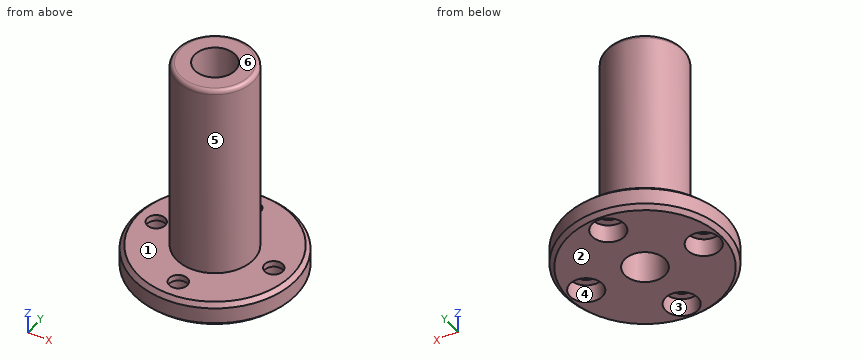
```python
from build123d import *

# Parameters (mm, degrees)
F0_R     = 20
F0_R_2   = 2.25
F0_R_3   = 5
F1_DEPTH = 6
F2_R     = 9.5
F2_R_2   = 5
F3_DEPTH = 49
F4_R     = 4
F5_DEPTH = 4.5
F6_SIZE  = 1
F7_R     = 1


with BuildPart() as f1:
    # F0 (on Top) → F1 (new body)
    with BuildSketch(Plane.XY):
        Circle(F0_R)
        with Locations((0, -14.5)):
            Circle(F0_R_2, mode=Mode.SUBTRACT)
        with Locations((-14.5, 0)):
            Circle(F0_R_2, mode=Mode.SUBTRACT)
        Circle(F0_R_3, mode=Mode.SUBTRACT)
        with Locations((14.5, 0)):
            Circle(F0_R_2, mode=Mode.SUBTRACT)
        with Locations((0, 14.5)):
            Circle(F0_R_2, mode=Mode.SUBTRACT)
    extrude(amount=F1_DEPTH)

    # F2 (on face) → F3 (join)
    with BuildSketch(Plane.XY.offset(6)):
        Circle(F2_R)
        Circle(F2_R_2, mode=Mode.SUBTRACT)
    extrude(amount=F3_DEPTH)

    # F4 (on face) → F5 (cut)
    with BuildSketch(Plane(origin=(0, 0, 0), x_dir=(1, 0, 0), z_dir=(0, 0, -1))):
        with Locations((0, 14.5)):
            Circle(F4_R)
        with Locations((14.5, 0)):
            Circle(F4_R)
        with Locations((0, -14.5)):
            Circle(F4_R)
        with Locations((-14.5, 0)):
            Circle(F4_R)
    extrude(amount=-F5_DEPTH, mode=Mode.SUBTRACT)

    # F6
    f6_edges = [f1.edges().sort_by_distance(p)[0] for p in [
        (-20, 0, 0),
        (-20, 0, 6),
    ]]
    chamfer(f6_edges, length=F6_SIZE)

    # F7
    f7_edges = [f1.edges().sort_by_distance(p)[0] for p in [
        (-9.5, 0, 55),
    ]]
    fillet(f7_edges, radius=F7_R)


solid = f1.part
```
Work out the finished part from the listing and answer in its coordinate system (mm). Face numbers are marked on the shaded views. A direction names the side the tool comes from. Coordinates: 2 decimals unless noted, no trailing zeros. Loops run counter-clockwise (first coordinate to the right, second up) from the corner with the lowest first, then second, coordinate; pieces in that order, holes last. Notation, with made-up numbers: (8.25, 82.5) - (56.25, 82.5) arc R36 ccw to (56.25, 116.5) - close; hole circle Ø7 at (11.5, 89). An arc over 180 degrees is marked (long way). Use a Markdown table: item, result.
Item 1: The mould has two halves that part along X. Classify the marked faces 4, 5 and 6: +X half, -X half, draft (parallel to the pull), parting line (faces both ways), or undercut.
Evaluation:
| item | result |
|---|---|
| face 4 | undercut |
| face 5 | parting line |
| face 6 | draft |
Item 2: Find section A-A, the plane y = 0. State how many separate pieces and enclosed holes the cut face has, and give its area (3 significant figures).
Evaluation:
| item | result |
|---|---|
| separate pieces | 4 |
| enclosed holes | 0 |
| area | 533 mm2 |
Item 3: Given pin 1 Ø5 at (x, y) = (0, -14.5) entering from +Z; pin 2 Ø6 at (x, y) = (14.5, 0) entering from -Z; pin 3 Ø2 at (x, z) = (3, 30) entering from +Y, each flat-ended and moving along its own axis, determine where each tip first touches the part or whether it passes through.
Evaluation:
| item | result |
|---|---|
| pin 1 | stops at z = 6 |
| pin 2 | stops at z = 4.5 |
| pin 3 | stops at y = 9.29 |
Item 4: Find section B-B, the plane z = 35.5. Determine the outline of the cut face in (x, y).
Evaluation:
| item | result |
|---|---|
| outline | circle Ø19 at (0, 0); hole circle Ø10 at (0, 0) |
Item 5: Consider probe 1 along Y at (x, z) = (14.5, 2.1); probe 2 along Z at (x, y) = (-13, -7.5); probe 3 along Y at (x, z) = (0, 5.5). Determine where each line is inside the solid, lowest interval first. Write a range as from..to.
Evaluation:
| item | result |
|---|---|
| probe 1 | y = -13.77..-4, 4..13.77 |
| probe 2 | z = 0..6 |
| probe 3 | y = -19.5..-16.75, -12.25..-5, 5..12.25, 16.75..19.5 |
Item 6: For the marked faces 1, 2 and 3, determine the directions among +Z, -Z, +X, -X, +Y, -Y from which every point of the face is accessible in a straight line to the end or side of a thin tool.
Evaluation:
| item | result |
|---|---|
| face 1 | +Z |
| face 2 | -Z, +X, -X, +Y, -Y |
| face 3 | -Z |
